from build123d import *

# Parameters (mm, degrees)
SKETCH2_R            = 300
SKETCH2_R_2          = 40
BOSS_EXTRUDE10_DEPTH = 10
CHAMFER1_SIZE        = 1
SKETCH13_R           = 6
CUT_EXTRUDE1_DEPTH   = 7
CHAMFER2_SIZE        = 1
SKETCH14_R           = 4
CUT_EXTRUDE2_DEPTH   = 3


with BuildPart() as part:
    # Sketch2 → Boss-Extrude10 (new body)
    with BuildSketch(Plane(origin=(0, 0, 0), x_dir=(1, 0, 0), z_dir=(0, 1, 0))):
        with Locations(Location((0, 0, 0), (0, 0, 270))):
            Circle(SKETCH2_R)
        with Locations(Location((0, 0, 0), (0, 0, 270))):
            Circle(SKETCH2_R_2, mode=Mode.SUBTRACT)
        with Locations(Location((0, 250, 0), (0, 0, 270))):
            Circle(SKETCH2_R_2, mode=Mode.SUBTRACT)
        with Locations(Location((176.776695297, 176.776695297, 0), (0, 0, 270))):
            Circle(SKETCH2_R_2, mode=Mode.SUBTRACT)
        with Locations(Location((250, 0, 0), (0, 0, 270))):
            Circle(SKETCH2_R_2, mode=Mode.SUBTRACT)
        with Locations(Location((176.776695297, -176.776695297, 0), (0, 0, 270))):
            Circle(SKETCH2_R_2, mode=Mode.SUBTRACT)
        with Locations(Location((0, -250, 0), (0, 0, 270))):
            Circle(SKETCH2_R_2, mode=Mode.SUBTRACT)
        with Locations(Location((-176.776695297, -176.776695297, 0), (0, 0, 270))):
            Circle(SKETCH2_R_2, mode=Mode.SUBTRACT)
        with Locations(Location((-250, 0, 0), (0, 0, 270))):
            Circle(SKETCH2_R_2, mode=Mode.SUBTRACT)
        with Locations(Location((-176.776695297, 176.776695297, 0), (0, 0, 270))):
            Circle(SKETCH2_R_2, mode=Mode.SUBTRACT)
    extrude(amount=BOSS_EXTRUDE10_DEPTH)

    # Chamfer1
    chamfer1_edges = [part.edges().sort_by_distance(p)[0] for p in [
        (176.776695297, 10, -216.776695297),
        (250, 10, -40),
        (176.776695297, 10, 136.776695297),
        (0, 10, 210),
        (-176.776695297, 10, 136.776695297),
        (-250, 10, -40),
        (-176.776695297, 10, -216.776695297),
        (0, 10, -300),
        (0, 10, -290),
    ]]
    chamfer(chamfer1_edges, length=CHAMFER1_SIZE)

    # Sketch13 → Cut-Extrude1 (cut)
    with BuildSketch(Plane(origin=(0, 10, 0), x_dir=(1, 0, 0), z_dir=(0, 1, 0))):
        with Locations(Location((-61, 0, 0), (0, 0, 270))):
            Circle(SKETCH13_R)
        with Locations(Location((-43.133513652, 43.133513652, 0), (0, 0, 270))):
            Circle(SKETCH13_R)
        with Locations(Location((0, 61, 0), (0, 0, 270))):
            Circle(SKETCH13_R)
        with Locations(Location((43.133513652, 43.133513652, 0), (0, 0, 270))):
            Circle(SKETCH13_R)
        with Locations(Location((61, 0, 0), (0, 0, 270))):
            Circle(SKETCH13_R)
        with Locations(Location((43.133513652, -43.133513652, 0), (0, 0, 270))):
            Circle(SKETCH13_R)
        with Locations(Location((0, -61, 0), (0, 0, 270))):
            Circle(SKETCH13_R)
        with Locations(Location((-43.133513652, -43.133513652, 0), (0, 0, 270))):
            Circle(SKETCH13_R)
    extrude(amount=-CUT_EXTRUDE1_DEPTH, mode=Mode.SUBTRACT)

    # Chamfer2
    chamfer2_edges = [part.edges().sort_by_distance(p)[0] for p in [
        (-61, 10, -6),
        (-43.133513652, 10, -49.133513652),
        (0, 10, -67),
        (43.133513652, 10, -49.133513652),
        (61, 10, -6),
        (43.133513652, 10, 37.133513652),
        (0, 10, 55),
        (-43.133513652, 10, 37.133513652),
    ]]
    chamfer(chamfer2_edges, length=CHAMFER2_SIZE)

    # Sketch14 → Cut-Extrude2 (cut)
    with BuildSketch(Plane.XZ):
        with Locations(Location((-61, 0, 0), (0, 0, 270))):
            Circle(SKETCH14_R)
        with Locations(Location((-43.133513652, 43.133513652, 0), (0, 0, 270))):
            Circle(SKETCH14_R)
        with Locations(Location((0, 61, 0), (0, 0, 270))):
            Circle(SKETCH14_R)
        with Locations(Location((43.133513652, 43.133513652, 0), (0, 0, 270))):
            Circle(SKETCH14_R)
        with Locations(Location((61, 0, 0), (0, 0, 270))):
            Circle(SKETCH14_R)
        with Locations(Location((43.133513652, -43.133513652, 0), (0, 0, 270))):
            Circle(SKETCH14_R)
        with Locations(Location((0, -61, 0), (0, 0, 270))):
            Circle(SKETCH14_R)
        with Locations(Location((-43.133513652, -43.133513652, 0), (0, 0, 270))):
            Circle(SKETCH14_R)
    extrude(amount=-CUT_EXTRUDE2_DEPTH, mode=Mode.SUBTRACT)


solid = part.part
The model under review builds one solid part; all positions refer to its coordinate system, in mm. Coordinates: 2 decimals unless noted, no trailing zeros. Put each result on its own line as item: value. Start each with the question number.
Q1. Add section A-A (y = 7.25). Count the separate pieces of the cut face and the enclosed holes in it, and give its area (3 significant figures).
Q2. Wall thickness on line 1 (X direction, y = 9.25, z = -201.5); line 2 (Z direction, x = -183, y = 2.5); line 3 (Z direction, x = 174, y = 9.75): over which ranges is each line inside the solid? List them lowest first.
Q3. The part is to be moulded in two halves that separate along X. For faces 1 (the cylindrical face through (-289.05, 4.44, -8.67)), 2 (the cylindrical face through (210.505, 4.437, 198.28)), 3 (the flat face through (71, 10, -4)), say which applies: +X half, -X half, draft (parallel to the pull), parting line (faces both ways), or undercut.
Q4. Clearance check with flat-ended pins moving along their axes: pin 1 (9.5 mm diameter, centred on x = 0, z = 61, fed in from +Y); pin 2 (6.5 mm diameter, centred on x = 43.13, z = 43.13, fed in from +Y); pin 3 (1.5 mm diameter, centred on y = 3, z = 165.5, fed in from -X). State where each tip first meets the part, or that it passes through.
Answers:
1. separate pieces: 1
1. enclosed holes: 17
1. area: 237,000 mm^2
2. line 1: x = -221.92 to -208.54, -145.01 to 145.01, 208.54 to 221.92
2. line 2: z = -237.72 to -216.29, -137.26 to 137.26, 216.29 to 237.72
2. line 3: z = -243.46 to -217.43, -136.12 to 136.12, 217.43 to 243.46
3. face 1: undercut
3. face 2: undercut
3. face 3: draft
4. pin 1: stops at y = 3
4. pin 2: passes through
4. pin 3: stops at x = -250.71
